Part model, mm, in its own coordinate system. A direction names the side the tool comes from. Give positions to 0.01 mm unless a question says otherwise; leave off trailing zeros. Loops run counter-clockwise (first coordinate to the right, second up) from the corner with the lowest first, then second, coordinate; pieces in that order, holes last. Notation, with made-up numbers: M 58.25,24 L 113.25,24 A11 ccw 113.25,42 Z; hole C -22.5,5.25 d4. An arc over 180 degrees is marked long. Answer in a Markdown table with one row per item.
from build123d import *

# Parameters (mm, degrees)
F0_W     = 2
F0_H     = 8
F0_W_2   = 35
F0_H_2   = 10
F1_DEPTH = 40
F2_DEPTH = 39
F3_R     = 4
F4_R     = 0.99999
F5_R     = 6


# Not quite as in the source:
# - a fillet or chamfer is up to 0.001 mm smaller than in the source, because OpenCascade refuses the exact size


with BuildPart() as f1:
    # F0 (on Top) → F1 (new body)
    with BuildSketch(Plane.XY):
        Polygon((40.35, -15), (55.35, -15), (55.35, 15), (40.35, 15), (40.35, 1.2), (40.35, -1), (41.35, -1), (41.35, -3), (40.35, -3), (40.35, -13), align=None)
        Polygon((42.35, -13), (42.35, 1.2), (42.35, 13), (53.35, 13), (53.35, -13), align=None, mode=Mode.SUBTRACT)
        Polygon((-55.35, -15), (40.35, -15), (40.35, -13), (1.15, -13), (-0.85, -13), (-12.35, -13), (-16.35, -13), (-51.35, -13), (-55.35, -13), align=None)
        Polygon((-12.35, -1), (-12.35, 1.2), (-16.35, 1.2), (-16.35, -0.8), (-15.35, -0.8), (-15.35, -3), (-16.35, -3), (-16.35, -13), (-12.35, -13), (-12.35, -3), (-13.35, -3), (-13.35, -1), align=None)
        Polygon((-55.35, 1.2), (-55.35, -13), (-51.35, -13), (-51.35, -3), (-52.35, -3), (-52.35, -0.8), (-51.35, -0.8), (-51.35, 1.2), align=None)
        with Locations((0.15, -9)):
            Rectangle(F0_W, F0_H)
        with Locations((-33.85, -8)):
            Rectangle(F0_W_2, F0_H_2)
        with BuildLine():
            Line((1.15, -13), (40.35, -13))
            Line((40.35, -13), (40.35, -3))
            Line((40.35, -3), (33.35, -3))
            Line((33.35, -3), (33.35, -5.5))
            ThreePointArc((33.35, -5.5), (30.85, -8), (28.35, -5.5))
            Line((28.35, -5.5), (28.35, -3))
            Line((28.35, -3), (-12.35, -3))
            Line((-12.35, -3), (-12.35, -13))
            Line((-12.35, -13), (-0.85, -13))
            Line((-0.85, -13), (-0.85, -5))
            Line((-0.85, -5), (1.15, -5))
            Line((1.15, -5), (1.15, -13))
        make_face()
    extrude(amount=F1_DEPTH)

    # F0 (on Top) → F2 (cut)
    with BuildSketch(Plane.XY):
        with Locations((-33.85, -8)):
            Rectangle(F0_W_2, F0_H_2)
        with BuildLine():
            Line((1.15, -13), (40.35, -13))
            Line((40.35, -13), (40.35, -3))
            Line((40.35, -3), (33.35, -3))
            Line((33.35, -3), (33.35, -5.5))
            ThreePointArc((33.35, -5.5), (30.85, -8), (28.35, -5.5))
            Line((28.35, -5.5), (28.35, -3))
            Line((28.35, -3), (-12.35, -3))
            Line((-12.35, -3), (-12.35, -13))
            Line((-12.35, -13), (-0.85, -13))
            Line((-0.85, -13), (-0.85, -5))
            Line((-0.85, -5), (1.15, -5))
            Line((1.15, -5), (1.15, -13))
        make_face()
    extrude(amount=F2_DEPTH, mode=Mode.SUBTRACT)

    # F3
    f3_edges = [f1.edges().sort_by_distance(p)[0] for p in [
        (42.35, -13, 20),
        (53.35, -13, 20),
        (53.35, 13, 20),
        (42.35, 13, 20),
        (-55.35, -15, 20),
    ]]
    fillet(f3_edges, radius=F3_R)

    # F4 (radius 1 in the source; OpenCascade refuses exactly that, so slightly less here)
    f4_edges = [f1.edges().sort_by_distance(p)[0] for p in [
        (40.35, -13, 19.5),
        (-0.85, -13, 19.5),
        (-0.85, -5, 19.5),
        (-16.35, -13, 19.5),
        (-16.35, 1.2, 20),
        (-12.35, 1.2, 20),
        (-55.35, 1.2, 20),
        (-51.35, 1.2, 20),
        (-51.35, -13, 19.5),
        (1.15, -5, 19.5),
        (1.15, -13, 19.5),
        (-12.35, -13, 19.5),
        (33.35, -3, 39.5),
        (28.35, -3, 39.5),
    ]]
    fillet(f4_edges, radius=F4_R)

    # F5
    f5_edges = [f1.edges().sort_by_distance(p)[0] for p in [
        (40.35, 15, 20),
        (55.35, 15, 20),
        (55.35, -15, 20),
    ]]
    fillet(f5_edges, radius=F5_R)


solid = f1.part
(1) Pull direction Y, two halves, no side cores. Call faces 1 (the face through (52.209, 11.797, 20.28)), 2 (the face through (40.35, 4, 20)), 3 (the face through (30.9, -8, 39.5)): +Y half, -Y half, draft (parallel to the pull), parting line (faces both ways), or undercut.
Recorded:
| item | result |
|---|---|
| face 1 | undercut |
| face 2 | draft |
| face 3 | +Y half |
(2) Saw through at B-B (x = 30.85). Write the cut outline in (y, z).
Recorded:
| item | result |
|---|---|
| outline | M -15,0 L -13,0 L -13,39 L -8,39 L -8,40 L -15,40 Z |
(3) Drill centre lines: line 1 along X through (y, z) = (-6.5, 11); line 2 along X through (y, z) = (-3.5, 6). Where is each one in solid material? Low to high.
Recorded:
| item | result |
|---|---|
| line 1 | x = -55.35 to -51.35, -16.35 to -12.35, -0.85 to 1.15, 40.35 to 42.35, 53.35 to 55.35 |
| line 2 | x = -55.35 to -51.35, -16.35 to -12.35, 40.35 to 42.35, 53.35 to 55.35 |
(4) Which spindle directions (+Z, -Z, +X, -X, +Y, -Y) get a long thin tool onto all of the face, cutting with end or side? Do faces 4 (the face through (48, 13, 20)), 5 (the face through (-14, 1.2, 20)), 6 (the face through (-12.35, -7, 19)). Say none if no direction does.
Recorded:
| item | result |
|---|---|
| face 4 | +Z, -Z |
| face 5 | +Z, -Z, -X, +Y |
| face 6 | -Z, +Y |
(5) Saw through at A-A (y = 5.5). Write the cut outline in (x, z), plus the area to 3 significant figures.
Recorded:
| item | result |
|---|---|
| outline | M 40.35,0 L 42.35,0 L 42.35,40 L 40.35,40 Z; M 53.35,0 L 55.35,0 L 55.35,40 L 53.35,40 Z |
| area | 160 mm^2 |
(6) Pin check, flat tips, straight feed: pin 1 Ø5 at (x, y) = (16, -9) entering from -Z; pin 2 Ø3 at (x, z) = (-28, 34.5) entering from +Y; pin 3 Ø6 at (y, z) = (4, 29) entering from -X; pin 4 Ø10 at (x, y) = (-44, 4.5) entering from +Z. Stop position of each tip, or through.
Recorded:
| item | result |
|---|---|
| pin 1 | stops at z = 39 |
| pin 2 | stops at y = -13 |
| pin 3 | stops at x = -54.95 |
| pin 4 | passes through |
